Autodesk Inventor part; units mm, degrees
ref_plane "YZ Plane" through (0, 0, 0) normal (1, 0, 0) x (0, 1, 0)
ref_plane "XZ Plane" through (0, 0, 0) normal (0, 1, 0) x (-1, 0, 0)
ref_plane "XY Plane" through (0, 0, 0) normal (0, 0, 1) x (1, 0, 0)
sketch "草圖1" plane through (0, 0, 0) normal (0, 1, 0) x (-1, 0, 0)
  line L0 (0, 0) -> (9, 0)
  line L1 (9, 0) -> (9, -198.5)
  line L2 (9, -198.5) -> (0, -198.5)
  line L3 (0, -198.5) -> (0, 0)
  line L4 (7, 0) -> (2, 0)
  line L5 (2, 0) -> (2, 9)
  line L6 (2, 9) -> (7, 9)
  line L7 (7, 9) -> (7, 0)
  line L8 (7, -198.5) -> (2, -198.5)
  line L9 (2, -198.5) -> (2, -207.5)
  line L10 (2, -207.5) -> (7, -207.5)
  line L11 (7, -207.5) -> (7, -198.5)
  point P0 (4.5, 0)
  point P1 (4.5, -198.5)
  dimension "d0" = 198.5
  dimension "d1" = 9
  dimension "d2" = 9
  dimension "d3" = 5
  dimension "d4" = 9
  dimension "d5" = 5
extrude "擠出1" add sketch "草圖1" along normal blind 3
properties part number "side_Bar" material "MDF Medium Density Fiberboard"
Input: part model. Units: mm. Frame: model coordinates. Round coordinates to 2 decimals unless told otherwise and drop trailing zeros. Order: outer loops, then holes, each group sorted by start corner. A loop starts at its lowest first (then second) coordinate and runs counter-clockwise, first axis right, second up. Notation, with made-up numbers: (59.25, -36.5) - (112.25, -36.5) arc R4 cw to (112.25, -32.5) - close; hole circle Ø5 at (45.25, -33.5). An arc over 180 degrees is marked (long way). Answer as a JSON object with one key per item and string values. Group by question number.
(1) Pin query (flat end, axial travel): P1, Ø0.6, axis at x = -1.5, y = 1.5, coming from the -Z side; P2, Ø1.5, axis at y = 2, z = -203.5, coming from the -X side; P3, Ø0.9, axis at y = 2, z = 6.5, coming from the +X side. Return the tip coordinate at first contact, or that it passes through.
(2) Cut plane A-A (y = 1.15). Return loops of the section in (x, z).
(3) Material intervals for probe 1 along Z at (x, y) = (-0.75, 2.65), sorted ascending. Write a range as from..to.
Here are the results:
{
 "1": {"P1": "stops at z = -198.5", "P2": "stops at x = -7", "P3": "stops at x = -2"},
 "2": {"outline": "(-9, -198.5) - (-7, -198.5) - (-7, -207.5) - (-2, -207.5) - (-2, -198.5) - (0, -198.5) - (0, 0) - (-2, 0) - (-2, 9) - (-7, 9) - (-7, 0) - (-9, 0) - close"},
 "3": {"probe 1": "z = -198.5..0"}
}
